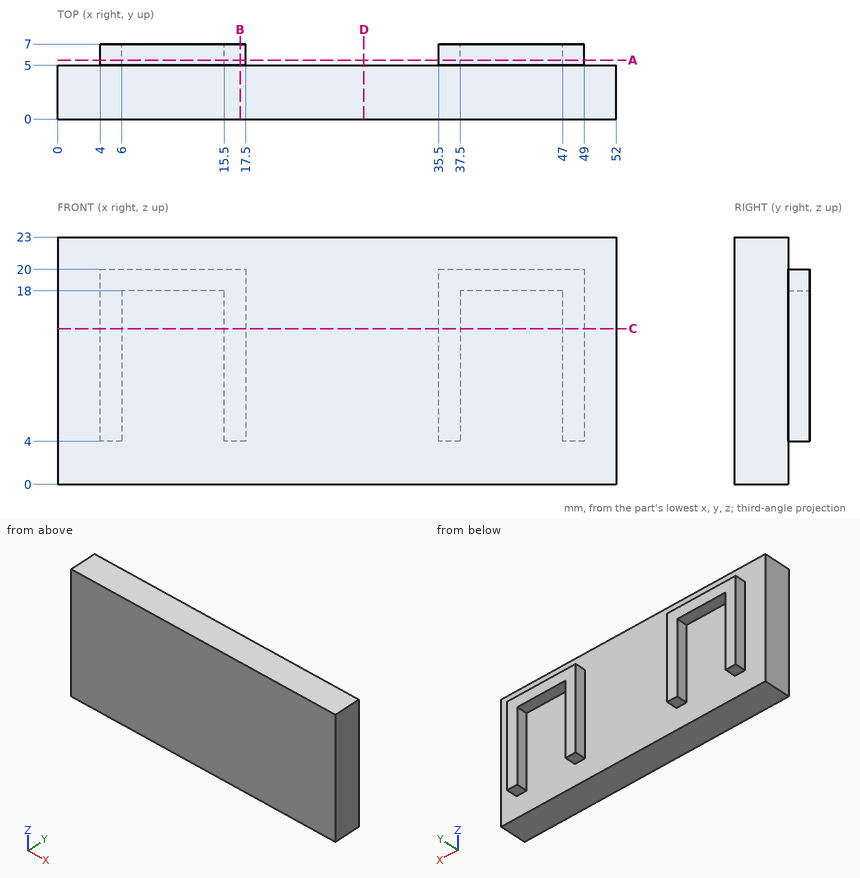
Job drawing, mm, ordinate dimensions from the low corner. One solid piece. Coordinates: 2 decimals unless noted, no trailing zeros. Write each loop counter-clockwise with the first axis right and the second up, starting at its lowest first coordinate (ties: lowest second). Pieces come first, ordered by that corner, then holes.
Item 1: Slice it at C-C (z = 14.5). Write the cut outline in (x, y), and give its area (3 significant figures).
Item 2: Slice it at A-A (y = 5.5). Write the cut outline in (x, z), and give its area (3 significant figures).
Item 3: Probe line 1 (X direction, y = 6.75, z = 12); line 2 (X direction, y = 5.75, z = 19.25); line 3 (Y direction, x = 8, z = 11.75). List the from-to ranges inside material, lowest first.
Item 4: Slice it at B-B (x = 17). Write the cut outline in (y, z), and give its area (3 significant figures).
Item 5: Pin check, flat tips, straight feed: pin 1 (1.5 mm diameter, centred on x = 7, z = 13, fed in from +Y); pin 2 (10 mm diameter, centred on x = 28, z = 5.5, fed in from -Y); pin 3 (0.6 mm diameter, centred on y = 6.5, z = 13.5, fed in from +X); pin 4 (0.6 mm diameter, centred on y = 6, z = 9.5, fed in from -X). Stop position of each tip, or through.
Item 6: Slice it at D-D (x = 28.5). Write the cut outline in (y, z).
Results found:
1. outline: (0, 0) - (52, 0) - (52, 5) - (49, 5) - (49, 7) - (47, 7) - (47, 5) - (37.5, 5) - (37.5, 7) - (35.5, 7) - (35.5, 5) - (17.5, 5) - (17.5, 7) - (15.5, 7) - (15.5, 5) - (6, 5) - (6, 7) - (4, 7) - (4, 5) - (0, 5) - close
1. area: 276 mm2
2. outline: (4, 4) - (6, 4) - (6, 18) - (15.5, 18) - (15.5, 4) - (17.5, 4) - (17.5, 20) - (4, 20) - close; (35.5, 4) - (37.5, 4) - (37.5, 18) - (47, 18) - (47, 4) - (49, 4) - (49, 20) - (35.5, 20) - close
2. area: 166 mm2
3. line 1: x = 4 to 6, 15.5 to 17.5, 35.5 to 37.5, 47 to 49
3. line 2: x = 4 to 17.5, 35.5 to 49
3. line 3: y = 0 to 5
4. outline: (0, 0) - (5, 0) - (5, 4) - (7, 4) - (7, 20) - (5, 20) - (5, 23) - (0, 23) - close
4. area: 147 mm2
5. pin 1: stops at y = 5
5. pin 2: stops at y = 0
5. pin 3: stops at x = 49
5. pin 4: stops at x = 4
6. outline: (0, 0) - (5, 0) - (5, 23) - (0, 23) - close
